Geometry check sheet. Reference: drawing and pictorial views, mm from the part's lowest x, y, z. A direction names the side the tool comes from. Round coordinates to 2 decimals unless told otherwise and drop trailing zeros. Write each loop counter-clockwise with the first axis right and the second up, starting at its lowest first coordinate (ties: lowest second). Pieces come first, ordered by that corner, then holes. Notation, with made-up numbers: M 23.5,44.5 L 47.5,44.5 A18 ccw 47.5,52.5 Z; hole C -12.5,21 d9. An arc over 180 degrees is marked long. Put each result on its own line as item: value. Start each with the question number.
(1) Section check B-B on x = 25. Count the separate pieces of the cut face and the enclosed holes in it, then the cut area to 3 significant figures.
(2) Mould release check, pull along Y, two halves, no side actions. Record for the marked faces 1, 2 and 3: pulls with the +Y half, pulls with the -Y half, needs draft (parallel to the pull), parting line crosses it, or undercut.
(3) Section check A-A on z = 37. Record the cut outline in (x, y).
(4) Tool access check on the marked faces 4 and 5. Record the directions out of +Z, -Z, +X, -X, +Y, -Y that give a thin tool (end or side, any length) a straight path to the whole face; none if there is none.
(5) Section check C-C on y = 64.5. Record the cut outline in (x, z), then the cut area to 3 significant figures.
(6) Gauge pin test, flat ends, axial feed: pin 1 (16 mm diameter, centred on x = 25, z = 37, fed in from +Y); pin 2 (9 mm diameter, centred on y = 107.5, z = 23.5, fed in from +X); pin 3 (1.3 mm diameter, centred on x = 96, z = 2.5, fed in from -Y); pin 4 (8 mm diameter, centred on x = 33.5, y = 31, fed in from +Z). Record the tip position at first contact, or that the pin passes through.
(7) Section check D-D on z = 28. Record the cut outline in (x, y).
(8) Material ranges on probe 1 along Y at (x, z) = (74, 28); probe 2 along Z at (x, y) = (25, 2.65); probe 3 along Z at (x, y) = (25, 2), recorded low to high.
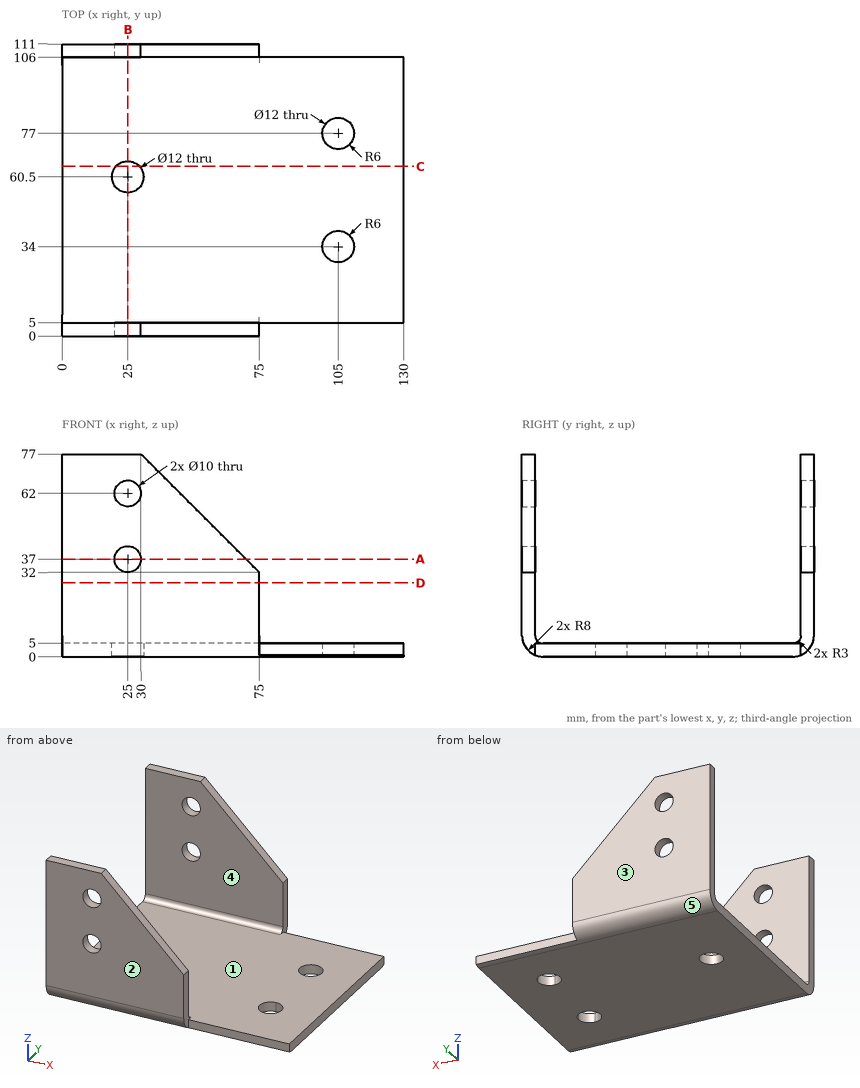
Answers follow:
1. separate pieces: 6
1. enclosed holes: 0
1. area: 991 mm^2
2. face 1: undercut
2. face 2: pulls with the -Y half
2. face 3: pulls with the +Y half
3. outline: M 0,0 L 20,0 L 20,5 L 0,5 Z; M 0,106 L 20,106 L 20,111 L 0,111 Z; M 30,0 L 70,0 L 70,5 L 30,5 Z; M 30,106 L 70,106 L 70,111 L 30,111 Z
4. face 4: +Z, +X, -X
4. face 5: -Z, +X, -X, +Y
5. outline: M 0,0 L 20.53,0 L 20.53,5 L 0,5 Z; M 29.47,0 L 130,0 L 130,5 L 29.47,5 Z
5. area: 605 mm^2
6. pin 1: stops at y = 111
6. pin 2: stops at x = 75
6. pin 3: stops at y = 5
6. pin 4: stops at z = 5
7. outline: M 0,0 L 75,0 L 75,5 L 0,5 Z; M 0,106 L 75,106 L 75,111 L 0,111 Z
8. probe 1: y = 0 to 5, 106 to 111
8. probe 2: z = 2.05 to 32, 42 to 57, 67 to 77
8. probe 3: z = 2.71 to 32, 42 to 57, 67 to 77
